```python
from build123d import *

# Parameters (mm, degrees)
BOSS_EXTRUDE1_DEPTH     = 6.0625
CUT_EXTRUDE1_DEPTH      = 24.31195039566617
CUT_EXTRUDE1_DEPTH_BACK = 24.31195039566617
SKETCH3_R               = 3.3782


with BuildPart() as part:
    # Sketch2 → Boss-Extrude1 (new, symmetric)
    with BuildSketch(Plane.XY):
        with BuildLine():
            Line((-14.25, 6.590447632748479), (-14.25, 12.344999999999999))
            ThreePointArc((-14.25, 12.344999999999999), (-12.762102448427667, 15.937102448427664), (-9.170000000000002, 17.425000000000004))
            Line((-9.170000000000002, 17.425000000000004), (9.36e-15, 17.425))
            Line((9.36e-15, 17.425), (9.169999999999998, 17.424999999999997))
            ThreePointArc((9.169999999999998, 17.424999999999997), (12.762102448427658, 15.937102448427659), (14.25, 12.344999999999999))
            Line((14.25, 12.344999999999999), (14.249999999999998, 6.5904476327484804))
            ThreePointArc((14.249999999999998, 6.5904476327484804), (13.659677420444995, 5.848038807835043), (12.80335731414868, 6.255920514699297))
            ThreePointArc((12.80335731414868, 6.255920514699297), (7.547040236593919, 12.087377038350068), (9.54e-15, 14.25))
            ThreePointArc((9.54e-15, 14.25), (-7.547040236593908, 12.087377038350072), (-12.803357314148682, 6.255920514699296))
            ThreePointArc((-12.803357314148682, 6.255920514699296), (-13.659677420444993, 5.848038807835042), (-14.25, 6.590447632748479))
        make_face()
    extrude(amount=BOSS_EXTRUDE1_DEPTH, both=True)

    # Sketch3 → Cut-Extrude1 (cut, two sides: drawn at the far end of the back side and taken through both)
    with BuildSketch(Plane(origin=(0, 0, 0), x_dir=(1, 0, 0), z_dir=(0, 1, 0)).offset(-CUT_EXTRUDE1_DEPTH_BACK)):
        with Locations(Location((0, 0, 0), (0, 0, 90))):
            Circle(SKETCH3_R)
    extrude(amount=CUT_EXTRUDE1_DEPTH + CUT_EXTRUDE1_DEPTH_BACK, mode=Mode.SUBTRACT)


solid = part.part
```
The listing builds one solid part. Answer for the finished solid, in the listing's coordinates (mm). Give positions to 0.01 mm unless a question says otherwise; leave off trailing zeros. Loops run counter-clockwise (first coordinate to the right, second up) from the corner with the lowest first, then second, coordinate; pieces in that order, holes last. Notation, with made-up numbers: M -39,-18.75 L 10,-18.75 A7 ccw 10,-5.75 Z; hole C 57.25,-8.75 d1. An arc over 180 degrees is marked long. One line per item, written item: value.
1. Section C-C on y = 11.5 is taken. Determine the outline of the cut face in (x, z).
Found:
outline: M -14.25,-6.06 L -8.42,-6.06 L -8.42,6.06 L -14.25,6.06 Z; M 8.42,-6.06 L 14.25,-6.06 L 14.25,6.06 L 8.42,6.06 Z
2. For a pull along X with two mould halves and no side action, classify faces 1 (the face through (-13.646, 5.845, 0.085)), 2 (the face through (0, 16, 6.062)), 3 (the face through (-12.8, 15.9, 0.1)) as pulls with the +X half, pulls with the -X half, needs draft (parallel to the pull), parting line crosses it, or undercut.
Found:
face 1: undercut
face 2: needs draft
face 3: pulls with the -X half
3. Each of these flat-tipped pins is pushed along its axis until it touches: P1, Ø5, axis at y = 16, z = 0, coming from the -X side; P2, Ø6, axis at x = 9, z = -2.5, coming from the -Y side. Where does it stop, or does it pass through?
Found:
P1: x = -14.12
P2: y = 7.69
4. Find the intervals of material crossed by probe 1 along X at (y, z) = (15.5, -2.75); probe 2 along X at (y, z) = (15.2, 0); probe 3 along Y at (x, z) = (8.5, 4.75) (3 decimals), in increasing order.
Found:
probe 1: -13.15 to -1.96, 1.96 to 13.15
probe 2: -13.37 to -3.38, 3.38 to 13.37
probe 3: 11.437 to 17.425
5. Section D-D on z = 3.75 is taken. Determine the outline of the cut face in (x, y) (3 decimals), plus the area to 3 significant figures.
Found:
outline: M -14.25,6.59 A0.762 ccw -12.803,6.256 A14.25 cw 12.803,6.256 A0.762 ccw 14.25,6.59 L 14.25,12.345 A5.08 ccw 9.17,17.425 L -9.17,17.425 A5.08 ccw -14.25,12.345 Z
area: 161 mm^2
6. Section A-A on z = 0 is taken. Determine the outline of the cut face in (x, y) (3 decimals).
Found:
outline: M -14.25,6.59 A0.762 ccw -12.803,6.256 A14.25 cw -3.378,13.844 L -3.378,17.425 L -9.17,17.425 A5.08 ccw -14.25,12.345 Z; M 3.378,13.844 A14.25 cw 12.803,6.256 A0.762 ccw 14.25,6.59 L 14.25,12.345 A5.08 ccw 9.17,17.425 L 3.378,17.425 Z
